```python
from build123d import *

# Parameters (mm, degrees)
TROU_TARAUD_M31_D = 2.5
SKETCH4_W         = 0.7
SKETCH4_H         = 0.7


with BuildPart() as part:
    # Sketch1 → Revolve1 (revolve)
    with BuildSketch(Plane.XY):
        Polygon((-3.75, 0), (-3.75, 3), (-1.25, 3), (-1.25, 2.5), (3.75, 2.5), (3.75, 0), align=None)
    revolve(axis=Axis((0, 0, 0), (1, 0, 0)))

    # Trou taraudé M31 (through all)
    with Locations(Plane(origin=(3.75, 0, 0), x_dir=(0, 0, -1), z_dir=(1, 0, 0))):
        with Locations((0, 0)):
            Hole(TROU_TARAUD_M31_D / 2)

    # Sketch4 → Cut-Revolve1 (revolve, cut)
    with BuildSketch(Plane.XY):
        with Locations((-0.9, 2.65)):
            Rectangle(SKETCH4_W, SKETCH4_H)
    revolve(axis=Axis((-0.090346983, 0, 0), (1, 0, 0)), mode=Mode.SUBTRACT)


solid = part.part
```
Work out the finished part from the listing and answer in its coordinate system (mm). A direction names the side the tool comes from. Coordinates: 2 decimals unless noted, no trailing zeros. Order: outer loops, then holes, each group sorted by start corner. A loop starts at its lowest first (then second) coordinate and runs counter-clockwise, first axis right, second up. Notation, with made-up numbers: (-18.5, 45) - (30.5, 45) arc R19 ccw to (30.5, 64) - close; hole circle Ø8 at (-35, 70.25). An arc over 180 degrees is marked (long way). Answer as a JSON object with one key per item and string values.
1. Each of these flat-tipped pins is pushed along its axis until it touches: P1, Ø2, axis at x = 3, z = 2, coming from the +Y side; P2, Ø3, axis at x = 0.5, z = -1, coming from the +Y side; P3, Ø2, axis at y = 0, z = 0, coming from the -X side; P4, Ø3, axis at y = -0.5, z = -0.5, coming from the +X side. Where does it stop, or does it pass through?
Output values:
{"P1": "stops at y = 2.29", "P2": "stops at y = 2.5", "P3": "passes through", "P4": "stops at x = 3.75"}
2. Consider line 1 (X direction, y = 2.4, z = 0); line 2 (X direction, y = 2.5, z = 0.65); line 3 (Y direction, x = -3, z = 0.7). Determine where each line is inside the solid, lowest interval first.
Output values:
{"line 1": "x = -3.75 to -1.25, -0.55 to 3.75", "line 2": "x = -3.75 to -1.25", "line 3": "y = -2.92 to -1.04, 1.04 to 2.92"}
3. Find section D-D on y = -1.85. Determine the outline of the cut face in (x, z).
Output values:
{"outline": "(-3.75, -2.36) - (-1.25, -2.36) - (-1.25, -1.37) - (-0.55, -1.37) - (-0.55, -1.68) - (3.75, -1.68) - (3.75, 1.68) - (-0.55, 1.68) - (-0.55, 1.37) - (-1.25, 1.37) - (-1.25, 2.36) - (-3.75, 2.36) - close"}
4. Find section C-C on x = -3. Determine the outline of the cut face in (y, z).
Output values:
{"outline": "circle Ø6 at (0, 0); hole circle Ø2.5 at (0, 0)"}
5. A tool of negligible diameter and unlimited length cuts with its end or side. For faces 4 (the face through (1.63, -0.54, -2.44)), 5 (the face through (-2, -3, 0)), 6 (the face through (-0.895, -1.825, -1.4)), from which of +Z, -Z, +X, -X, +Y, -Y can it reach the whole face along a straight path? Write none if from no direction.
Output values:
{"face 4": "+X", "face 5": "+X, -X", "face 6": "none"}
6. Find section A-A on z = 0. Determine the outline of the cut face in (x, y).
Output values:
{"outline": "(-3.75, -3) - (-1.25, -3) - (-1.25, -2.3) - (-0.55, -2.3) - (-0.55, -2.5) - (3.75, -2.5) - (3.75, -1.25) - (-3.75, -1.25) - close; (-3.75, 1.25) - (3.75, 1.25) - (3.75, 2.5) - (-0.55, 2.5) - (-0.55, 2.3) - (-1.25, 2.3) - (-1.25, 3) - (-3.75, 3) - close"}
7. The mould has two halves that part along X. Classify faces 1 (the face through (-3.75, -1, -1)), 2 (the face through (3.75, 1, 1)), 3 (the face through (-1.25, 2, -2)): +X half, -X half, draft (parallel to the pull), parting line (faces both ways), or undercut.
Output values:
{"face 1": "-X half", "face 2": "+X half", "face 3": "undercut"}
